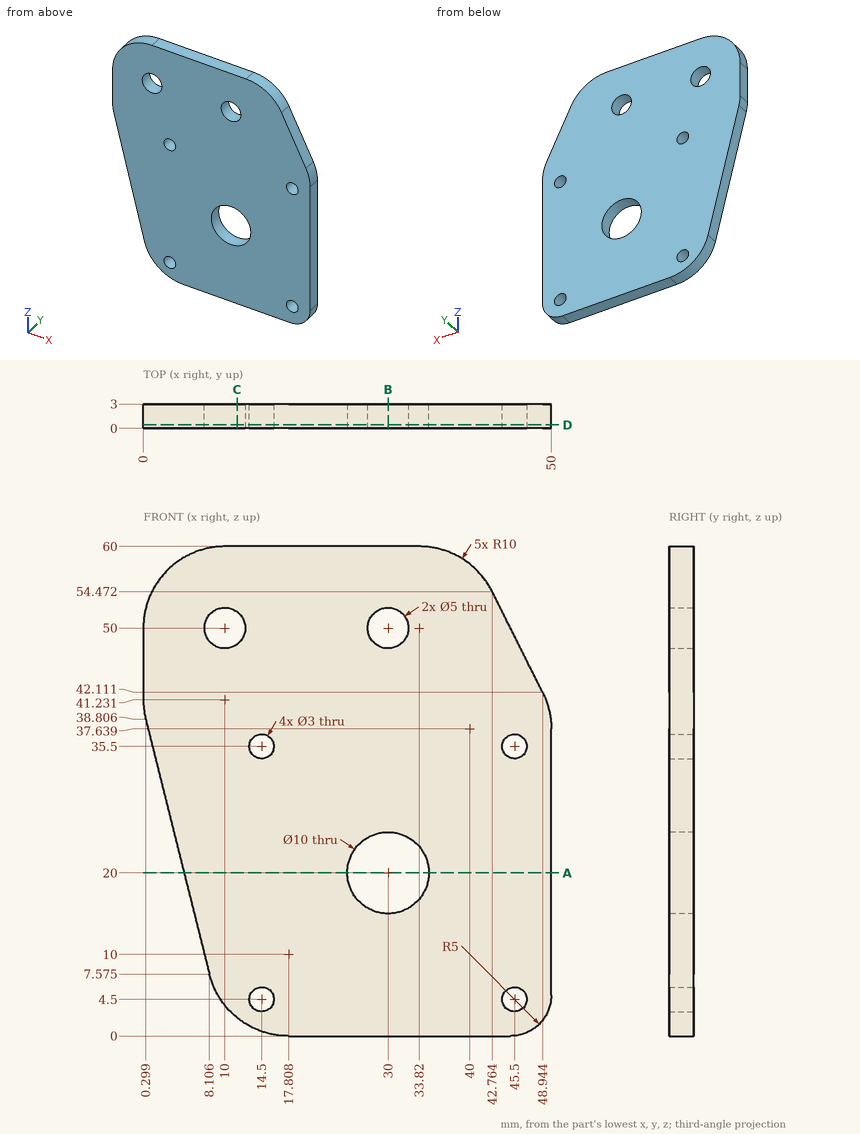
Study the drawing (mm; zero at the part's minimum x, y, z) and answer. Give positions to 0.01 mm unless a question says otherwise; leave off trailing zeros. Order: outer loops, then holes, each group sorted by start corner. A loop starts at its lowest first (then second) coordinate and runs counter-clockwise, first axis right, second up. Notation, with made-up numbers: (46.5, 9) - (81.5, 9) arc R25 cw to (81.5, 26) - close; hole circle Ø9 at (44, 74). An arc over 180 degrees is marked (long way). Answer in a Markdown table with one row per item. Add a question column.
Q1. Given P1, Ø2.5, axis at x = 45.5, z = 35.5, coming from the +Y side, flat-ended and moving along its own axis, determine where the tip first touches the part or whether it passes through.
Q2. The part is cut by section A-A (z = 20). Determine the outline of the cut face in (x, y), then the cut area to 3 significant figures.
Q3. The part is cut by section D-D (y = 0.45). Determine the outline of the cut face in (x, z) (1 decimal), then the cut area to 3 significant figures.
Q4. The part is cut by section C-C (x = 11.5). Determine the outline of the cut face in (y, z).
Q5. Find the intervals of material crossed by line 1 along X through (y, z) = (0.9, 50); line 2 along Z through (x, y) = (30, 2.45); line 3 along X through (y, z) = (1.3, 20), in increasing order. Write a range as [from, to].
Q6. The part is cut by section B-B (x = 30). Determine the outline of the cut face in (y, z).
Determined:
| question | item | result |
|---|---|---|
| 1 | P1 | passes through |
| 2 | outline | (5, 0) - (25, 0) - (25, 3) - (5, 3) - close; (35, 0) - (50, 0) - (50, 3) - (35, 3) - close |
| 2 | area | 105 mm² |
| 3 | outline | (0, 41.2) arc R10 ccw to (0.3, 38.8) - (8.1, 7.6) arc R10 ccw to (17.8, 0) - (45, 0) arc R5 ccw to (50, 5) - (50, 37.6) arc R10 ccw to (48.9, 42.1) - (42.8, 54.5) arc R10 ccw to (33.8, 60) - (10, 60) arc R10 ccw to (0, 50) - close; hole circle Ø5 at (10, 50); hole circle Ø3 at (14.5, 4.5); hole circle Ø3 at (14.5, 35.5); hole circle Ø10 at (30, 20); hole circle Ø5 at (30, 50); hole circle Ø3 at (45.5, 4.5); hole circle Ø3 at (45.5, 35.5) |
| 3 | area | 2,510 mm² |
| 4 | outline | (0, 2.24) - (3, 2.24) - (3, 48) - (0, 48) - close; (0, 52) - (3, 52) - (3, 60) - (0, 60) - close |
| 5 | line 1 | x = [0, 7.5], [12.5, 27.5], [32.5, 45] |
| 5 | line 2 | z = [0, 15], [25, 47.5], [52.5, 60] |
| 5 | line 3 | x = [5, 25], [35, 50] |
| 6 | outline | (0, 0) - (3, 0) - (3, 15) - (0, 15) - close; (0, 25) - (3, 25) - (3, 47.5) - (0, 47.5) - close; (0, 52.5) - (3, 52.5) - (3, 60) - (0, 60) - close |
